Autodesk Fusion 360 part; units mm, degrees
sketch "Sketch1" plane through (0, 0, 0) normal (1, 0, 0) x (0, 1, 0)
  circle A0 centre (0, 0) radius 0.5
  line L0 (0.325, -0.325) -> (-0.325, -0.325)
  line L1 (-0.325, -0.325) -> (-0.325, 0.325)
  line L2 (-0.325, 0.325) -> (0.325, 0.325)
  line L3 (0.325, 0.325) -> (0.325, -0.325)
  line L4 (0.325, -0.325) -> (-0.325, 0.325) construction
  line L5 (-0.325, -0.325) -> (0.325, 0.325) construction
  dimension "d1" = 1
  dimension "d2" = 0.65
  dimension "d3" = 0.65
extrude "Extrude1" add sketch "Sketch1" along normal blind 43 contours A0 | L0 L1 L2 L3
sketch "Sketch2" plane through (43, 0, 0) normal (1, 0, 0) x (0, 1, 0)
  circle A0 centre (0, 0) radius 0.5
  line L0 (0.325, -0.325) -> (-0.325, -0.325)
  line L1 (-0.325, -0.325) -> (-0.325, 0.325)
  line L2 (-0.325, 0.325) -> (0.325, 0.325)
  line L3 (0.325, 0.325) -> (0.325, -0.325)
  line L4 (0.325, -0.325) -> (-0.325, 0.325) construction
  line L5 (-0.325, -0.325) -> (0.325, 0.325) construction
  dimension "d8" = 0.65
  dimension "d9" = 0.65
extrude "Extrude2" add sketch "Sketch2" along normal blind 1.685 contours L0 L1 L2 L3
extrude "Extrude3" add sketch "Sketch1" against normal blind 1.685 contours L0 L1 L2 L3
sketch "Sketch3" plane through (0, 0, -0.325) normal (0, 0, -1) x (1, 0, 0)
  line L0 (43, 0.325) -> (43, -0.325)
  line L1 (43, -0.325) -> (44.685, -0.325)
  line L2 (44.685, -0.325) -> (44.685, 0.325)
  line L3 (44.685, 0.325) -> (43, 0.325)
  line L4 (44.685, 0.325) -> (44.035, 0.325)
  line L5 (44.035, 0.325) -> (44.035, -0.325)
  line L6 (44.035, -0.325) -> (44.685, -0.325)
  line L7 (44.685, -0.325) -> (44.685, 0.325)
  line L8 (44.685, 0.325) -> (44.035, -0.325) construction
  line L9 (44.035, 0.325) -> (44.685, -0.325) construction
  point P0 (44.36, 0)
  dimension "d14" = 0.65
  dimension "d15" = 0.65
sketch "Sketch4" plane through (0, 0, -0.325) normal (0, 0, -1) x (1, 0, 0)
  line L0 (0, -0.325) -> (0, 0.325)
  line L1 (0, 0.325) -> (-1.685, 0.325)
  line L2 (-1.685, 0.325) -> (-1.685, -0.325)
  line L3 (-1.685, -0.325) -> (0, -0.325)
  line L4 (-1.035, -0.325) -> (-1.685, -0.325)
  line L5 (-1.685, -0.325) -> (-1.685, 0.325)
  line L6 (-1.685, 0.325) -> (-1.035, 0.325)
  line L7 (-1.035, 0.325) -> (-1.035, -0.325)
  line L8 (-1.035, -0.325) -> (-1.685, 0.325) construction
  line L9 (-1.685, -0.325) -> (-1.035, 0.325) construction
  point P0 (-1.36, 0)
  dimension "d17" = 0.65
  dimension "d18" = 0.65
extrude "Extrude4" add sketch "Sketch4" sketch "Sketch3" along normal blind 2.75 contours L1 L2 L3 L4 L5 L6 L7 of sketch 2 contours L1 L2 L3 L4 L5 L6 L7
fillet "Fillet1" radius 0.5 2 edges at (-1.035, 0, -0.325) (44.035, 0, -0.325)
fillet "Fillet2" radius 1 2 edges at (-1.685, 0, 0.325) (44.685, 0, 0.325)
fillet "Fillet3" radius 0.2 32 edges at (-1.36, -0.325, -3.075) (-1.035, 0, -3.075) (-1.36, 0.325, -3.075) (-1.685, 0, -3.075) (-0.8886, -0.325, -0.4714) (-1.035, -0.325, -1.95) (-0.2675, -0.325, -0.325) (-0.3425, -0.325, 0.325) (-1.3921, -0.325, 0.0321) (-1.685, -0.325, -1.875) (-0.3425, 0.325, 0.325) (-1.3921, 0.325, 0.0321) (-1.685, 0.325, -1.875) (-0.8886, 0.325, -0.4714) (-0.2675, 0.325, -0.325) (-1.035, 0.325, -1.95) (43.3425, -0.325, 0.325) (44.3921, -0.325, 0.0321) (44.685, -0.325, -1.875) (44.035, -0.325, -1.95) (43.8886, -0.325, -0.4714) (43.2675, -0.325, -0.325) (44.685, 0.325, -1.875) (44.3921, 0.325, 0.0321) (43.3425, 0.325, 0.325) (43.8886, 0.325, -0.4714) (44.035, 0.325, -1.95) (43.2675, 0.325, -0.325) (44.36, 0.325, -3.075) (44.685, 0, -3.075) (44.36, -0.325, -3.075) (44.035, 0, -3.075)
equation "d1 = width"
equation "d2 = d3"
equation "d3 = d1 * 0.65"
equation "width = 1 mm"
equation "baseLenght = 43 mm"
equation "d6 = baseLenght"
equation "d8 = width * 0.65"
equation "d9 = d8"
equation "d14 = width * 0.65"
equation "d15 = d14"
equation "d17 = width * 0.65"
equation "d18 = d17"
equation "d26 = 0.2 * width"
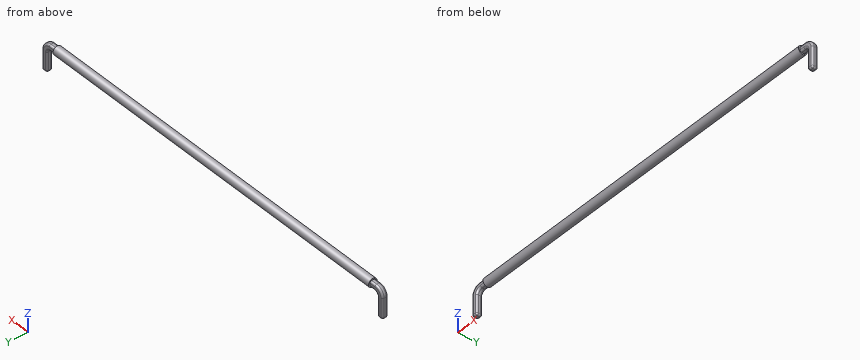
CAD build for the part. Positions are in the model's coordinates, mm. Round coordinates to 2 decimals unless told otherwise and drop trailing zeros. Loops run counter-clockwise (first coordinate to the right, second up) from the corner with the lowest first, then second, coordinate; pieces in that order, holes last. Notation, with made-up numbers: M -4,10 L 35,10 A33 cw 35,40 Z; hole C -26,7.25 d4. An arc over 180 degrees is marked long. Use a Markdown table: item, result. Add a question column.
(1) Drill centre lines: line 1 (X direction, y = -0.05, z = -1) (3 decimals); line 2 (X direction, y = -0.3, z = 0.3); line 3 (X direction, y = -0.25, z = -0.8). Where is each one in solid material? Low to high.
(2) Cut at A-A (z = -1.45). Give the cut face in (x, y) (3 decimals), and give its area (3 significant figures).
(3) Cut at B-B (x = 3). Give the cut face in (y, z), and give its area (3 significant figures).
(4) Flat gauge pins, fed straight in: pin 1 (0.7 mm diameter, centred on x = 44, z = -1.5, fed in from -Y) (3 decimals); pin 2 (0.7 mm diameter, centred on x = -1, z = -1.5, fed in from +Y) (3 decimals). Where does each tip first touch, or does it go through?
Geometry says:
| question | item | result |
|---|---|---|
| 1 | line 1 | x = -1.685 to -1.035, 44.035 to 44.685 |
| 1 | line 2 | x = 0 to 43 |
| 1 | line 3 | x = -1.64 to -1.08, 44.08 to 44.64 |
| 2 | outline | M -1.685,-0.125 A0.2 ccw -1.485,-0.325 L -1.235,-0.325 A0.2 ccw -1.035,-0.125 L -1.035,0.125 A0.2 ccw -1.235,0.325 L -1.485,0.325 A0.2 ccw -1.685,0.125 Z; M 44.035,-0.125 A0.2 ccw 44.235,-0.325 L 44.485,-0.325 A0.2 ccw 44.685,-0.125 L 44.685,0.125 A0.2 ccw 44.485,0.325 L 44.235,0.325 A0.2 ccw 44.035,0.125 Z |
| 2 | area | 0.776 mm² |
| 3 | outline | C 0,0 d1 |
| 3 | area | 0.785 mm² |
| 4 | pin 1 | stops at y = -0.325 |
| 4 | pin 2 | stops at y = 0.325 |
